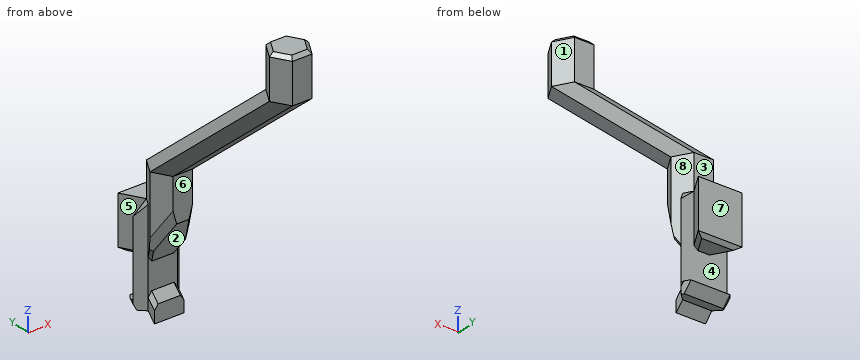
from build123d import *
from OCP.BRepFilletAPI import BRepFilletAPI_MakeChamfer

# Parameters (mm, degrees)
BOSS_EXTRUDE1_DEPTH      = 25.4
BOSS_EXTRUDE2_DEPTH      = 12.7
BOSS_EXTRUDE3_DEPTH      = 15.239999999999998
CHAMFER1_SIZE            = 7.46
CHAMFER1_SIZE2           = 12.540000000000001
BOSS_EXTRUDE4_DEPTH      = 12.7
BOSS_EXTRUDE5_DEPTH      = 24.384
BOSS_EXTRUDE6_DEPTH      = 4.265467
BOSS_EXTRUDE6_DEPTH_BACK = 4.265467
BOSS_EXTRUDE7_DEPTH      = 6.704137
BOSS_EXTRUDE7_DEPTH_BACK = 6.704137
CHAMFER2_SIZE            = 3.556
CHAMFER3_SIZE            = 1.016
CHAMFER3_SIZE2           = 2.1468318359684853
CHAMFER3_SIZE2_2         = 0.7623750143993072


with BuildPart() as part:
    # Sketch1 → Boss-Extrude1 (new body)
    with BuildSketch(Plane.XY):
        Polygon((5.715, 0), (2.8574999999999884, 4.949335182628073), (-2.857500000000022, 4.949335182628053), (-5.715, -3.991e-14), (-2.8574999999999533, -4.949335182628093), (2.8575000000000577, -4.949335182628033), align=None)
    extrude(amount=BOSS_EXTRUDE1_DEPTH)



with BuildPart() as body_2:
    # Sketch2 → Boss-Extrude2 (new body)
    with BuildSketch(Plane.XY.offset(63.5)):
        Polygon((-2.8574999999999533, -49.399335182628086), (2.8575000000000577, -49.399335182628036), (5.714999999999993, -44.45000000000016), (2.8574999999999884, -39.50066481737193), (-2.857500000000022, -39.50066481737194), (-5.715, -44.45000000000003), align=None)
    extrude(amount=BOSS_EXTRUDE2_DEPTH)


with BuildPart() as part_1:
    add(part.part)

    add(body_2.part)  # loft1 joins it to this body
    # loft from a face of the part (loft1)
    loft([part_1.faces().sort_by_distance((4.1e-15, -1.66e-15, 25.4))[0], part_1.faces().sort_by_distance((2.71e-15, -44.45000000000001, 63.5))[0]])

    # Sketch4 → Boss-Extrude3 (add)
    with BuildSketch(Plane(origin=(0, 0, 0), x_dir=(-1, 0, 0), z_dir=(0, 0, -1))):
        Polygon((2.857500000000022, 4.949335182628053), (6.3770272409799595, 11.045335182628051), (-6.377027240979914, 11.04533518262805), (-2.8574999999999884, 4.949335182628073), align=None)
    extrude(amount=-BOSS_EXTRUDE3_DEPTH)

    # Chamfer1
    chamfer1_edges = [part_1.edges().sort_by_distance(p)[0] for p in [
        (5.196e-14, -4.949335182628063, 0),
    ]]
    chamfer1_side = [part_1.faces().sort_by_distance(p)[0] for p in [
        (-7.04e-15, 3.3439435440816787, 0),
    ]]
    chamfer(chamfer1_edges, length=CHAMFER1_SIZE, length2=CHAMFER1_SIZE2, reference=chamfer1_side[0])

    # Sketch5 → Boss-Extrude4 (add)
    with BuildSketch(Plane(origin=(0, 0, 0), x_dir=(-1, 0, 0), z_dir=(0, 0, -1))):
        Polygon((-2.8574999999999884, 4.949335182628073), (2.857500000000022, 4.949335182628053), (4.265466991845397, 2.510664817371916), (-4.265466991845346, 2.5106648173720054), align=None)
    extrude(amount=BOSS_EXTRUDE4_DEPTH)

    # Sketch6 → Boss-Extrude5 (add)
    with BuildSketch(Plane(origin=(0, 0, -12.7), x_dir=(-1, 0, 0), z_dir=(0, 0, -1))):
        Polygon((-4.265466991845346, 2.5106648173720054), (-6.7041373571014065, 4.949335182628073), (-2.8574999999999884, 4.949335182628073), (2.857500000000022, 4.949335182628053), (6.7041373571013665, 4.949335182628074), (4.265466991845397, 2.510664817371916), align=None)
    extrude(amount=-BOSS_EXTRUDE5_DEPTH)

    # Sketch7 → Boss-Extrude6 (add, two sides: drawn at the far end of the back side and taken through both)
    with BuildSketch(Plane(origin=(0, 0, 0), x_dir=(0, 0, -1), z_dir=(1, 0, 0)).offset(-BOSS_EXTRUDE6_DEPTH_BACK)):
        Polygon((7.765575597798472, 2.5106648173720054), (10.159999999999973, 2.5106648173720054), (12.7, 2.5106648173720054), (15.094424402201499, 0.11624041517056517), (10.159999999999973, 0.11624041517056455), align=None)
    extrude(amount=BOSS_EXTRUDE6_DEPTH + BOSS_EXTRUDE6_DEPTH_BACK)

    # Sketch7<3> → Boss-Extrude7 (add, two sides: drawn at the far end of the back side and taken through both)
    with BuildSketch(Plane(origin=(0, 0, 0), x_dir=(0, 0, -1), z_dir=(1, 0, 0)).offset(-BOSS_EXTRUDE7_DEPTH_BACK)):
        Polygon((10.159999999999972, 7.489335182628074), (10.159999999999972, 4.949335182628073), (12.7, 4.949335182628073), align=None)
    extrude(amount=BOSS_EXTRUDE7_DEPTH + BOSS_EXTRUDE7_DEPTH_BACK)

    # Chamfer2
    # the kernel refuses this chamfer: 3.556 mm, written as the material it adds along each edge
    with BuildSketch(Plane(origin=(8.837919344448796, -5.409054972524991, 11.684000000000001), x_dir=(-0.023812127644090044, -0.013747938305293153, 0.9996219169112966), z_dir=(-0.500000000000001, 0.866025403784438, 0))) as chamfer2_piece_1_section:
        Polygon((CHAMFER2_SIZE * 0.999621916911, CHAMFER2_SIZE * 0.0274958766106), (-CHAMFER2_SIZE * 0.0274958766106, CHAMFER2_SIZE * 0.999621916911), (0, 0), align=None)
    chamfer2_piece_1 = extrude(amount=21.10574339410437, mode=Mode.PRIVATE)
    chamfer2_piece_1 = split(chamfer2_piece_1, bisect_by=Plane(origin=(5.0850917452486755, 3.330289570775337, 13.032835155075794), z_dir=(-0.7071067811865487, 0.7071067811865465, 0)), keep=Keep.TOP, mode=Mode.PRIVATE)
    chamfer2_piece_1 = split(chamfer2_piece_1, bisect_by=Plane(origin=(4.3712108447170275, 4.9493351826280785, 13.032835155075794), z_dir=(3.57e-15, -1, 0)), keep=Keep.TOP, mode=Mode.PRIVATE)
    add(chamfer2_piece_1)
    with BuildSketch(Plane(origin=(1.7149523526033228, 12.869054972524992, 11.684000000000001), x_dir=(0.023812127644090457, -0.013747938305293174, 0.9996219169112966), z_dir=(-0.4999999999999951, -0.8660254037844415, 0))) as chamfer2_piece_2_section:
        Polygon((CHAMFER2_SIZE * 0.999621916911, CHAMFER2_SIZE * 0.0274958766106), (-CHAMFER2_SIZE * 0.0274958766106, CHAMFER2_SIZE * 0.999621916911), (0, 0), align=None)
    chamfer2_piece_2 = extrude(amount=21.10574339410434, mode=Mode.PRIVATE)
    chamfer2_piece_2 = split(chamfer2_piece_2, bisect_by=Plane(origin=(-4.371210844717055, 4.949335182628047, 13.032835155075803), z_dir=(3.57e-15, -1, 0)), keep=Keep.TOP, mode=Mode.PRIVATE)
    chamfer2_piece_2 = split(chamfer2_piece_2, bisect_by=Plane(origin=(-5.085091745248726, 3.330289570775309, 13.032835155075805), z_dir=(0.7071067811865749, 0.7071067811865203, 0)), keep=Keep.TOP, mode=Mode.PRIVATE)
    add(chamfer2_piece_2)

    # Chamfer3: one chamfer whose edges measure the first distance from different faces: ONE call of the kernel's chamfer builder (chamfer() names one face for all edges)
    chamfer3_edges_1 = [part_1.edges().sort_by_distance(p)[0] for p in [
        (-4.265467, 1.3134526162712852, -8.962787798899223),
        (4.265467, 1.3134526162712852, -8.962787798899223),
        (-4.617263620489991, 7.997335182628052, 0),
        (-2.309e-14, 11.045335182628051, 0),
        (4.617263620489951, 7.997335182628062, 0),
        (-6.704137, 6.219335182628074, -11.429999999999986),
        (6.704137, 6.219335182628074, -11.429999999999986),
        (5.196e-14, -49.399335182628064, 76.2),
        (-4.286249999999977, -46.92466759131406, 76.2),
        (4.286250000000026, -46.9246675913141, 76.2),
        (-4.286250000000011, -41.975332408685986, 76.2),
        (4.28624999999999, -41.97533240868604, 76.2),
        (-1.688e-14, -39.500664817371934, 76.2),
    ]]
    chamfer3_edges_2 = [part_1.edges().sort_by_distance(p)[0] for p in [
        (-4.286249999999978, -2.4746675913140663, 8.380170027469429),
        (4.286250000000031, -2.4746675913140157, 8.380170027469497),
    ]]
    chamfer3_side_2 = [part_1.faces().sort_by_distance(p)[0] for p in [
        (1.357e-14, -0.9394076954343201, 5.7994516502132),
    ]]
    chamfer3_edges_3 = [part_1.edges().sort_by_distance(p)[0] for p in [
        (-4.990233495922706, 1.255332408685926, 2.1101700274694246),
        (4.990233495922681, 1.2553324086859914, 2.1101700274694926),
    ]]
    chamfer3_side_3 = [part_1.faces().sort_by_distance(p)[0] for p in [
        (1.357e-14, -0.9394076954343201, 5.7994516502132),
    ]]
    chamfer3 = BRepFilletAPI_MakeChamfer(part_1.part.solid().wrapped)
    for e in chamfer3_edges_1:
        chamfer3.Add(CHAMFER3_SIZE, e.wrapped)
    for e in chamfer3_edges_2:
        chamfer3.Add(CHAMFER3_SIZE, CHAMFER3_SIZE2, e.wrapped, chamfer3_side_2[0].wrapped)  # the first distance lies on this face
    for e in chamfer3_edges_3:
        chamfer3.Add(CHAMFER3_SIZE, CHAMFER3_SIZE2_2, e.wrapped, chamfer3_side_3[0].wrapped)  # the first distance lies on this face
    add(Compound.cast(chamfer3.Shape()), mode=Mode.REPLACE)


solid = part_1.part
Work out the finished part from the listing and answer in its coordinate system (mm). Face numbers are marked on the shaded views. A direction names the side the tool comes from. Round coordinates to 2 decimals unless told otherwise and drop trailing zeros. Write each loop counter-clockwise with the first axis right and the second up, starting at its lowest first coordinate (ties: lowest second). Pieces come first, ordered by that corner, then holes. Notation, with made-up numbers: (16.5, -15) -> (67.5, -15) arc R21 cw to (67.5, 18) -> close; hole circle Ø3 at (17, 14.25). An arc over 180 degrees is marked (long way). Answer as CSV lines item,"result". Start each with the question number.
(1) A tool of negligible diameter and unlimited length cuts with its end or side. For the marked faces 1, 2, 3, 4 and 5, from which of +Z, -Z, +X, -X, +Y, -Y can it reach the whole face along a straight path? Write none if from no direction.
(2) The part is cut by section A-A, the plane x = -0.25. Give the vertices of the cut face in (y, z).
(3) Find the intervals of material crossed by probe 1 along Y at (x, z) = (3, 2.5); probe 2 along Z at (x, y) = (1.25, 7); probe 3 along Y at (x, z) = (-6, 8), in increasing order.
(4) The part is cut by section B-B, the plane z = -1. Give the vertices of the cut face in (x, y).
(5) Each of these flat-tipped pins is pushed along its axis until it touches: pin 1 (2 mm diameter, centred on x = -2, z = 56.5, fed in from +Y); pin 2 (4 mm diameter, centred on x = 0, z = -12, fed in from -Y); pin 3 (0.7 mm diameter, centred on y = 1, z = -11.5, fed in from -X). Where does it stop, or does it pass through?
(6) The mould has two halves that part along Y. Classify the marked faces 6, 7 and 8: +Y half, -Y half, draft (parallel to the pull), parting line (faces both ways), or undercut.
Output values:
1,face 1,"+Z, +X, +Y"
1,face 2,"+X, -X, -Y"
1,face 3,"+Z, +X, -X, +Y"
1,face 4,"none"
1,face 5,"+Z, -X"
2,outline,"(-49.4, 63.5) -> (-4.95, 25.4) -> (-4.95, 12.54) -> (2.51, 0) -> (2.51, -7.77) -> (0.12, -10.16) -> (0.12, -15.09) -> (2.51, -12.7) -> (4.95, -12.7) -> (7.49, -10.16) -> (4.95, -10.16) -> (4.95, 0) -> (10.03, 0) -> (11.05, 1.02) -> (11.05, 15.24) -> (4.95, 15.24) -> (4.95, 25.4) -> (-39.5, 63.5) -> (-39.5, 75.18) -> (-40.52, 76.2) -> (-48.38, 76.2) -> (-49.4, 75.18) -> close"
3,probe 1,"y = 1.02 to 4.95, 5.2 to 11.05"
3,probe 2,"z = -10.65 to -10.16, 0 to 15.24"
3,probe 3,"y = 4.25 to 4.95, 10.39 to 11.05"
4,outline,"(-6.7, 4.95) -> (-4.27, 2.51) -> (4.27, 2.51) -> (6.7, 4.95) -> close"
5,pin 1,"stops at y = -30.17"
5,pin 2,"stops at y = 0.12"
5,pin 3,"stops at x = -4.27"
6,face 6,"-Y half"
6,face 7,"+Y half"
6,face 8,"undercut"
